```python
from build123d import *

# Parameters (mm, degrees)
F0_W     = 114.3
F0_H     = 50.8
F1_DEPTH = 88.9
F3_DEPTH = 25.4
F5_DEPTH = 25.4
F6_R     = 25.4
F7_DEPTH = 92.202


with BuildPart() as f1:
    # F0 (on Top) → F1 (new body)
    with BuildSketch(Plane.XY):
        with Locations((37.11038, -46.895293)):
            Rectangle(F0_W, F0_H)
    extrude(amount=F1_DEPTH)

    # F2 (on face) → F3 (cut)
    with BuildSketch(Plane.XZ.offset(72.295293)):
        Polygon((68.86038, 0), (94.26038, 0), (94.26038, 88.9), (18.62484, 88.9), align=None)
        Polygon((18.62484, 0), (68.86038, 0), (18.62484, 88.9), align=None)
    extrude(amount=-F3_DEPTH, mode=Mode.SUBTRACT)

    # F4 (on face) → F5 (join)
    with BuildSketch(Plane.XZ.offset(46.895293)):
        Polygon((78.006379, 0), (18.62484, 88.9), (18.62484, 0), align=None)
    extrude(amount=F5_DEPTH)

    # F6 (on face) → F7 (cut)
    with BuildSketch(Plane.XZ.offset(72.295293)):
        with Locations((36.774643, 43.852847)):
            Circle(F6_R)
    extrude(amount=-F7_DEPTH, mode=Mode.SUBTRACT)


solid = f1.part
```
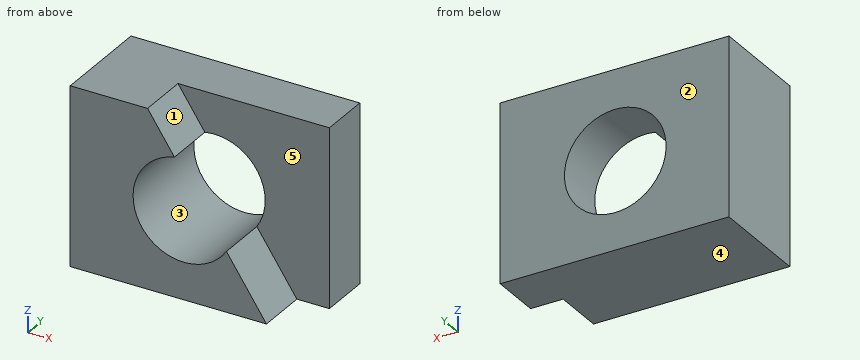
Verification items for the finished model (mm, model axes). Face numbers are marked on the shaded views. A direction names the side the tool comes from. Give positions to 0.01 mm unless a question says otherwise; leave off trailing zeros. Loops run counter-clockwise (first coordinate to the right, second up) from the corner with the lowest first, then second, coordinate; pieces in that order, holes last. Notation, with made-up numbers: M -33.75,10 L 15.25,10 A16 ccw 15.25,15 Z; hole C 43,60.5 d7. An arc over 180 degrees is marked long. One line per question, with ' | ' between items.
Item 1: Depth check by flat-ended pin: P1, Ø10, axis at x = 62, z = 38.5, coming from the -Y side; P2, Ø1, axis at x = 50.5, y = -50, coming from the +Z side. Enter the tip coordinate at first touch or a pass-through.
Completed:
P1: stops at y = -46.9 | P2: stops at z = 22.81
Item 2: Tool access check on the marked faces 4 and 5. Record the directions out of +Z, -Z, +X, -X, +Y, -Y that give a thin tool (end or side, any length) a straight path to the whole face; none if there is none.
Completed:
face 4: -Z, +X, -X, +Y, -Y | face 5: +Z, +X, -Y
Item 3: Section check C-C, the plane y = -65. Record the cut outline in (x, z).
Completed:
outline: M -20.04,0 L 78.01,0 L 58.02,29.93 A25.4 cw long 32.05,68.81 L 18.62,88.9 L -20.04,88.9 Z
Item 4: Thickness scan on line 1 (Y direction, x = 77.5, z = 79); line 2 (Z direction, x = 17, y = -61.5); line 3 (Z direction, x = 26.5, y = -41). Record the ranges inside material, lowest first. Write a range as [from, to].
Completed:
line 1: y = [-46.9, -21.5] | line 2: z = [0, 27.91], [59.79, 88.9] | line 3: z = [0, 20.62], [67.08, 88.9]
Item 5: Section check D-D, the plane y = -43.5. Record the cut outline in (x, z).
Completed:
outline: M -20.04,0 L 94.26,0 L 94.26,88.9 L -20.04,88.9 Z; hole C 36.77,43.85 d50.8
Item 6: Section check B-B, the plane z = 41. Record the cut outline in (x, y), plus the area to 3 significant figures.
Completed:
outline: M -20.04,-72.3 L 11.54,-72.3 L 11.54,-21.5 L -20.04,-21.5 Z; M 62.01,-46.9 L 94.26,-46.9 L 94.26,-21.5 L 62.01,-21.5 Z | area: 2,420 mm^2
Item 7: Draft check along X on the marked faces 1, 2 and 3. Enter one of: +X half, -X half, draft (parallel to the pull), parting line (faces both ways), or undercut.
Completed:
face 1: +X half | face 2: draft | face 3: undercut
Item 8: Section check A-A, the plane x = 16. Record the cut outline in (y, z), plus the area to 3 significant figures.
Completed:
outline: M -72.3,0 L -21.5,0 L -21.5,29.24 L -72.3,29.24 Z; M -72.3,58.47 L -21.5,58.47 L -21.5,88.9 L -72.3,88.9 Z | area: 3,030 mm^2
